Part model, mm, in its own coordinate system. A direction names the side the tool comes from. Round coordinates to 2 decimals unless told otherwise and drop trailing zeros. Write each loop counter-clockwise with the first axis right and the second up, starting at its lowest first coordinate (ties: lowest second). Pieces come first, ordered by that corner, then holes. Notation, with made-up numbers: (41.5, 72) -> (99.5, 72) arc R19 ccw to (99.5, 85) -> close; hole circle Ø3 at (72.25, 86). An arc over 180 degrees is marked (long way). Return JSON: item names as keys, results as strings. Group by question number.
(1) Saw through at B-B (x = -20). List the corners of the cut face in (y, z), plus the area to 3 significant figures.
(2) Saw through at D-D (z = 6.75). List the corners of the cut face in (x, y).
(3) Drop flat-ended pins along their axis: pin 1 Ø2.5 at (x, y) = (-20, 15) entering from -Z; pin 2 Ø1 at (x, y) = (-11, 10.5) entering from +Z; pin 3 Ø5 at (x, z) = (20, 2) entering from +Y; pin 4 Ø2 at (y, z) = (3.5, 3) entering from -X. Give the stop position or say it passes through.
(4) Saw through at A-A (z = 2). List the corners of the cut face in (x, y), plus the area to 3 significant figures.
(5) Tool access for faces 1 (the flat face through (0, 11, -13)), 2 (the flat face through (0, 13, -10)): list every direction of +Z, -Z, +X, -X, +Y, -Y with a clear straight run to the whole face (end or side of a thin tool).
(6) Drill centre lines: L1, parallel to X at y = 1.9, z = 2; L2, parallel to Y at x = 20, z = -11.15; L3, parallel to Z at x = 15, y = 12.5. Where is each one in solid material? Low to high. Write a range as from..to.
(7) Saw through at C-C (y = 15). List the corners of the cut face in (x, z), plus the area to 3 significant figures.
(8) Mould opens along Y. For faces 3 (the flat face through (0, 0, -2)), 4 (the cylindrical face through (21.5, 14.93, -11.48)), 5 (the flat face through (0, 3, 0)), 6 (the flat face through (-30, 1.3, -6.9)) say: +Y half, -Y half, draft (parallel to the pull), parting line (faces both ways), or undercut.
from build123d import *

# Parameters (mm, degrees)
SKETCH1_W           = 60
SKETCH1_H           = 20
BOSS_EXTRUDE1_DEPTH = 3
SKETCH3_W           = 60
SKETCH3_H           = 3
BOSS_EXTRUDE2_DEPTH = 23
FILLET2_R           = 1
SKETCH4_R           = 1.5
CUT_EXTRUDE1_DEPTH  = 39.327535793
SKETCH6_R           = 1.5
CUT_EXTRUDE2_DEPTH  = 43.766809561


with BuildPart() as part:
    # Sketch1 → Boss-Extrude1 (new body)
    with BuildSketch(Plane(origin=(0, 0, 0), x_dir=(1, 0, 0), z_dir=(0, 1, 0))):
        Rectangle(SKETCH1_W, SKETCH1_H)
    extrude(amount=BOSS_EXTRUDE1_DEPTH)

    # Sketch3 → Boss-Extrude2 (add)
    with BuildSketch(Plane(origin=(0, 0, 0), x_dir=(1, 0, 0), z_dir=(0, 1, 0))):
        with Locations((0, 11.5)):
            Rectangle(SKETCH3_W, SKETCH3_H)
    extrude(amount=BOSS_EXTRUDE2_DEPTH)

    # Fillet2
    fillet2_edges = [part.edges().sort_by_distance(p)[0] for p in [
        (0, 3, 10),
        (-30, 13, -10),
        (30, 13, -10),
        (0, 0, -13),
        (30, 11.5, -13),
        (-30, 11.5, -13),
        (30, 23, -11.5),
        (0, 23, -13),
        (-30, 3, 0),
        (-30, 23, -11.5),
        (0, 23, -10),
        (0, 3, -10),
        (-30, 0, -1.5),
        (0, 0, 10),
        (30, 0, -1.5),
        (-30, 1.5, 10),
        (30, 1.5, 10),
        (30, 3, 0),
    ]]
    fillet(fillet2_edges, radius=FILLET2_R)

    # Sketch4 → Cut-Extrude1 (cut, through all)
    with BuildSketch(Plane(origin=(0, 3, 0), x_dir=(1, 0, 0), z_dir=(0, 1, 0))):
        with Locations(Location((-20, -2, 0), (0, 0, 270))):
            Circle(SKETCH4_R)
        with Locations(Location((20, -2, 0), (0, 0, 90))):
            Circle(SKETCH4_R)
    extrude(amount=-CUT_EXTRUDE1_DEPTH, mode=Mode.SUBTRACT)

    # Sketch6 → Cut-Extrude2 (cut, through all)
    with BuildSketch(Plane.XY.offset(-10)):
        with Locations((-20, 15)):
            Circle(SKETCH6_R)
        with Locations(Location((20, 15, 0), (0, 0, 180))):
            Circle(SKETCH6_R)
    extrude(amount=-CUT_EXTRUDE2_DEPTH, mode=Mode.SUBTRACT)


solid = part.part
Computed values:
{
 "1": {"outline": "(0, -12) arc R1 ccw to (1, -13) -> (13.5, -13) -> (13.5, -10) -> (4, -10) arc R1 cw to (3, -9) -> (3, 0.5) -> (0, 0.5) -> close; (0, 3.5) -> (3, 3.5) -> (3, 9) arc R1 ccw to (2, 10) -> (1, 10) arc R1 ccw to (0, 9) -> close; (16.5, -13) -> (22, -13) arc R1 ccw to (23, -12) -> (23, -11) arc R1 ccw to (22, -10) -> (16.5, -10) -> close", "area": "110 mm2"},
 "2": {"outline": "(-30, 1) arc R1 ccw to (-29, 0) -> (29, 0) arc R1 ccw to (30, 1) -> (30, 2) arc R1 ccw to (29, 3) -> (-29, 3) arc R1 ccw to (-30, 2) -> close"},
 "3": {"pin 1": "through", "pin 2": "z = -10", "pin 3": "y = 3", "pin 4": "x = -29.87"},
 "4": {"outline": "(-30, 1) arc R1 ccw to (-29, 0) -> (-21.5, 0) -> (-21.5, 3) -> (-29, 3) arc R1 ccw to (-30, 2) -> close; (-18.5, 0) -> (18.5, 0) -> (18.5, 3) -> (-18.5, 3) -> close; (21.5, 0) -> (29, 0) arc R1 ccw to (30, 1) -> (30, 2) arc R1 ccw to (29, 3) -> (21.5, 3) -> close", "area": "161 mm2"},
 "5": {"face 1": "-Z, +X, -X, +Y, -Y", "face 2": "+Z, +X, -X, +Y"},
 "6": {"L1": "-30..-21.5, -18.5..18.5, 21.5..30", "L2": "0..13.5, 16.5..23", "L3": "-13..-10"},
 "7": {"outline": "(-30, -12) arc R1 ccw to (-29, -13) -> (-21.5, -13) -> (-21.5, -10) -> (-29, -10) arc R1 ccw to (-30, -11) -> close; (-18.5, -13) -> (18.5, -13) -> (18.5, -10) -> (-18.5, -10) -> close; (21.5, -13) -> (29, -13) arc R1 ccw to (30, -12) -> (30, -11) arc R1 ccw to (29, -10) -> (21.5, -10) -> close", "area": "161 mm2"},
 "8": {"face 3": "-Y half", "face 4": "undercut", "face 5": "+Y half", "face 6": "draft"}
}
